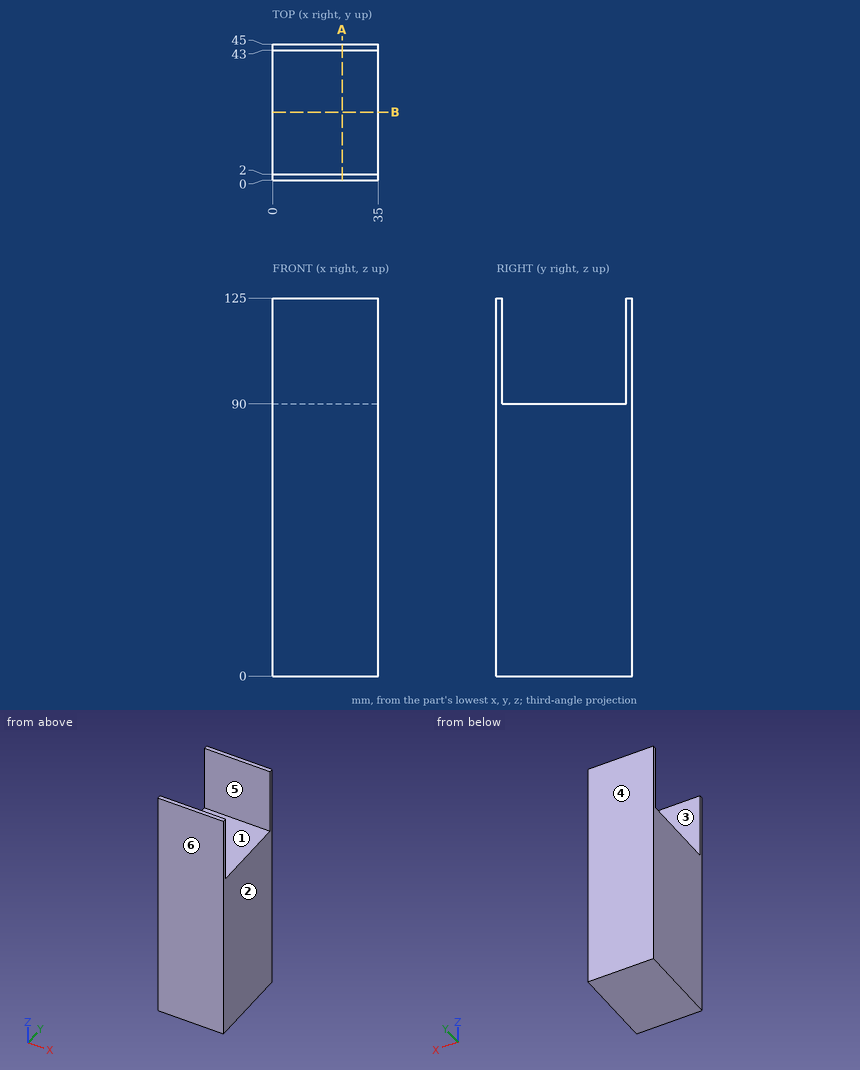
Input: dimensioned drawing with shaded views. Units: mm. Origin: part minimum x, y, z. A direction names the side the tool comes from. Coordinates: 2 decimals unless noted, no trailing zeros. Loops run counter-clockwise (first coordinate to the right, second up) from the corner with the lowest first, then second, coordinate; pieces in that order, holes last. Notation, with made-up numbers: M 89.25,-11 L 120.25,-11 A21 cw 120.25,-5 Z; hole C -38.5,-24 d8. An arc over 180 degrees is marked long. One line per item, written item: value.
(1) Section B-B (y = 22.5). Output: boundary loops of the cut face in (x, z).
Filled in:
outline: M 0,0 L 35,0 L 35,90 L 0,90 Z
(2) Line query: line 1 along Y through (x, z) = (26.5, 107); line 2 along Z through (x, y) = (33, 7). Output: solid intervals per line, ascending. Write a range as from..to.
Filled in:
line 1: 0..2, 43..45
line 2: 0..90
(3) Section A-A (x = 23). Output: boundary loops of the cut face in (y, z), and give its area (3 significant figures).
Filled in:
outline: M 0,0 L 45,0 L 45,125 L 43,125 L 43,90 L 2,90 L 2,125 L 0,125 Z
area: 4,190 mm^2
(4) Reachability of the marked faces 1 and 2 from +Z, -Z, +X, -X, +Y, -Y: full face, straight path, thin tool, end or side. Return the list, or none.
Filled in:
face 1: +Z, +X, -X
face 2: +Z, -Z, +X, +Y, -Y
(5) Pin query (flat end, axial travel): pin 1 (17.5 mm diameter, centred on x = 22.5, y = 17, fed in from +Z). Return the tip coordinate at first contact, or that it passes through.
Filled in:
pin 1: z = 90
(6) Pull-direction query (Y, two-part tool) for the marked faces 3, 4, 5 and 6; classes: +Y half, -Y half, draft (parallel to the pull), parting line (faces both ways), or undercut.
Filled in:
face 3: undercut
face 4: +Y half
face 5: undercut
face 6: -Y half
